Autodesk Inventor part; units mm, degrees
ref_plane "YZ Plane" through (0, 0, 0) normal (1, 0, 0) x (0, 1, 0)
ref_plane "XZ Plane" through (0, 0, 0) normal (0, 1, 0) x (-1, 0, 0)
ref_plane "XY Plane" through (0, 0, 0) normal (0, 0, 1) x (1, 0, 0)
sketch "Sketch1" plane through (0, 0, 0) normal (0, 0, 1) x (1, 0, 0)
  circle A0 centre (0, 0) radius 40
  circle A1 centre (0, 0) radius 41.5
  circle A2 centre (0, 0) radius 3.5
  circle A3 centre (0, 0) radius 5
  circle A4 centre (26, 0) radius 6.8
  circle A5 centre (26, 0) radius 7.8
  line L0 (0, 0) -> (43.8957, 0) construction
  line L1 (4.9183, 0.9) -> (18.2521, 0.9)
  line L2 (33.7479, 0.9) -> (39.9899, 0.9)
  line L3 (4.9183, -0.9) -> (18.2521, -0.9)
  line L4 (33.7479, -0.9) -> (39.9899, -0.9)
  line L5 (-4.9183, -0.9) -> (-18.2521, -0.9)
  line L6 (-4.9183, 0.9) -> (-18.2521, 0.9)
  circle A6 centre (-26, 0) radius 7.8
  circle A7 centre (-26, 0) radius 6.8
  line L7 (-33.7479, 0.9) -> (-39.9899, 0.9)
  line L8 (-33.7479, -0.9) -> (-39.9899, -0.9)
  line L9 (1.2333, -3.7857) -> (-1.2333, -3.7857)
  line L10 (-1.6333, -3.3857) -> (-1.6333, 3.3857)
  line L11 (-1.2333, 3.7857) -> (1.2333, 3.7857)
  line L12 (1.6333, 3.3857) -> (1.6333, -3.3857)
  line L13 (1.6333, -3.7857) -> (-1.6333, 3.7857) construction
  line L14 (-1.6333, -3.7857) -> (1.6333, 3.7857) construction
  arc A8 (-1.2333, 3.7857) -> (-1.6333, 3.3857) centre (-1.2333, 3.3857) ccw
  arc A9 (1.6333, 3.3857) -> (1.2333, 3.7857) centre (1.2333, 3.3857) ccw
  arc A10 (1.2333, -3.7857) -> (1.6333, -3.3857) centre (1.2333, -3.3857) ccw
  arc A11 (-1.6333, -3.3857) -> (-1.2333, -3.7857) centre (-1.2333, -3.3857) ccw
  line L15 (3.3857, -1.6333) -> (-3.3857, -1.6333)
  line L16 (-3.7857, -1.2333) -> (-3.7857, 1.2333)
  line L17 (-3.3857, 1.6333) -> (3.3857, 1.6333)
  line L18 (3.7857, 1.2333) -> (3.7857, -1.2333)
  line L19 (3.7857, -1.6333) -> (-3.7857, 1.6333) construction
  line L20 (-3.7857, -1.6333) -> (3.7857, 1.6333) construction
  arc A12 (-3.3857, 1.6333) -> (-3.7857, 1.2333) centre (-3.3857, 1.2333) ccw
  arc A13 (3.7857, 1.2333) -> (3.3857, 1.6333) centre (3.3857, 1.2333) ccw
  arc A14 (3.3857, -1.6333) -> (3.7857, -1.2333) centre (3.3857, -1.2333) ccw
  arc A15 (-3.7857, -1.2333) -> (-3.3857, -1.6333) centre (-3.3857, -1.2333) ccw
  point P0 (-4.9183, -0.9)
  point P1 (4.9183, -0.9)
  point P2 (-1.6333, -3.0955)
  point P3 (-1.6333, 3.0955)
  point P4 (1.6333, 3.0955)
  point P5 (1.6333, -3.0955)
  point P6 (-4.9183, 0.9)
  point P7 (-33.7479, 0.9)
  point P8 (-3.0955, -1.6333)
  point P9 (-3.0955, 1.6333)
  point P10 (3.0955, 1.6333)
  point P11 (3.0955, -1.6333)
  dimension "d0" = 80
  dimension "d3" = 10
  dimension "d1" = 83
  dimension "d2" = 7
  dimension "d4" = 13.6
  dimension "d5" = 26
  dimension "d6" = 15.6
  dimension "d10" = 0.9
  dimension "d11" = 0.9
  dimension "d14" = 360
  dimension "d16" = 7.5714
  dimension "d17" = 3.2667
  dimension "d18" = 0.4
  dimension "d29" = 7.5714
  dimension "d30" = 3.2667
  dimension "d31" = 0.4
extrude "Extrusion1" add sketch "Sketch1" along normal blind 5 contours A0 L4 A5 L2 | L7 A6 L8 A0 | A5 | A6 | A5 L3 A3 L1 | L6 A3 L5 A6 | A3 | A1
sketch "Sketch2" plane through (0, 0, 5) normal (0, 0, 1) x (1, 0, 0)
  arc A0 (33.7479, 0.9) -> (18.2521, 0.9) centre (26, 0) ccw
  circle A1 centre (26, 0) radius 7.7
  circle A2 centre (26, 0) radius 5.8
  arc A3 (18.2521, -0.9) -> (33.7479, -0.9) centre (26, 0) ccw
  circle A4 centre (-26, 0) radius 5.8
  circle A5 centre (-26, 0) radius 7.7
  point P0 (0, 0)
  point P1 (18.3528, 0.9)
  point P2 (33.6472, 0.9)
  point P3 (-18.2521, 0.9)
  point P4 (-33.7479, 0.9)
  point P5 (18.7723, -2.9327)
  dimension "d21" = 7.8
  dimension "d22" = 11.6
  dimension "d27" = 360
extrude "Extrusion2" add sketch "Sketch2" along normal blind 0.4
equation "\"d0\" = D_yttreRing_i"
equation "\"d3\" = D_axel + d_axelRing"
equation "\"d1\" = D_yttreRing_i + d_yttreRing"
equation "\"d2\" = D_axel"
equation "\"d4\" = D_magnet + d_toleransRing"
equation "\"d6\" = d_toleransRing + D_magnet + d_magnetHållarRing"
equation "\"d11\" = 0.5 * d_stöttor"
equation "\"d18\" = r_filletAxel"
equation "\"d31\" = r_filletAxel"
equation "\"d19\" = h_höjdMagnetRotor"
equation "\"d22\" = D_magnet - d_magnetSkydd"
equation "\"d23\" = h_magnetSkydd"
equation "\"D_yttreRing_i\" = 80"
equation "\"d_yttreRing\" = 3"
equation "\"D_magnet\" = 13"
equation "\"D_axel\" = 7"
equation "\"d_axelRing\" = 3"
equation "\"h_höjdMagnetRotor\" = 5"
equation "\"d_stöttor\" = 1.8"
equation "\"d_toleransRing\" = 0.6"
equation "\"d_magnetHållarRing\" = 2"
equation "\"l_magnetHållarRingFrånOrigo\" = 26"
equation "\"r_filletAxel\" = 0.4"
equation "\"h_magnetSkydd\" = 0.4"
equation "\"d_magnetSkydd\" = 1.4"
properties part number "Magnet_rotor_parametriserad_02"
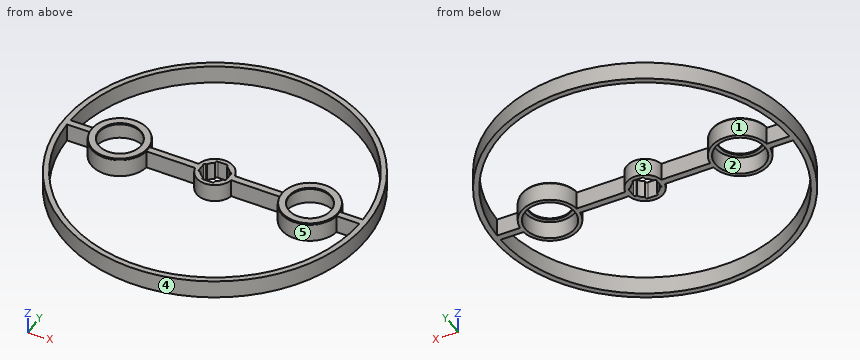
Read the model definition and answer for the solid it produces. Units are mm, in the model's axes. Face numbers are marked on the shaded views. A direction names the side the tool comes from. Round coordinates to 2 decimals unless told otherwise and drop trailing zeros. Order: outer loops, then holes, each group sorted by start corner. A loop starts at its lowest first (then second) coordinate and runs counter-clockwise, first axis right, second up.
1) The mould has two halves that part along X. Classify the marked faces 3, 4 and 5: released by +X, released by -X, zero draft, split by the parting line, or undercut.
2) For the marked faces 1 and 2, determine the directions among +Z, -Z, +X, -X, +Y, -Y from which every point of the face is accessible in a straight line to the end or side of a thin tool.
3) The part is cut by section C-C on x = 9. Write down the section's boundary in (y, z).
4) The part is cut by section B-B on y = -27. Write down the section's boundary in (x, z), plus the area to 3 significant figures.
5) Flat-ended cylindrical pins translate along their axes: pin 1 (1.5 mm diameter, centred on y = 26.5, z = 4.5, fed in from +X); pin 2 (2.5 mm diameter, centred on x = -8.5, z = 3.5, fed in from +Y); pin 3 (1.5 mm diameter, centred on x = 36.5, z = 3.5, fed in from +Y). Find the tip coordinate at first contact, or state that the pin passes through.
6) Straight lines are drawn through the part: L1, parallel to Y at x = -17.5, z = 1.25; L2, parallel to X at y = -7, z = 2.65; L3, parallel to Y at x = 26, z = 5.3. For each, find the intervals that lie inside material, in ascending order.
7) The part is cut by section D-D on y = -15. Write down the section's boundary in (x, z), plus the area to 3 significant figures.
8) The part is cut by section A-A on x = 0. Write down the section's boundary in (y, z), plus the area to 3 significant figures.
Resolved:
1. face 3: undercut
1. face 4: split by the parting line
1. face 5: undercut
2. face 1: +Z, -Z
2. face 2: -Z
3. outline: (-40.51, 0) - (-38.97, 0) - (-38.97, 5) - (-40.51, 5) - close; (-0.9, 0) - (0.9, 0) - (0.9, 5) - (-0.9, 5) - close; (38.97, 0) - (40.51, 0) - (40.51, 5) - (38.97, 5) - close
4. outline: (-31.52, 0) - (-29.51, 0) - (-29.51, 5) - (-31.52, 5) - close; (29.51, 0) - (31.52, 0) - (31.52, 5) - (29.51, 5) - close
4. area: 20.0 mm2
5. pin 1: stops at x = 32.55
5. pin 2: stops at y = 40.86
5. pin 3: stops at y = 21.08
6. L1: y = -37.63 to -35.97, -0.9 to 0.9, 35.97 to 37.63
6. L2: x = -40.91 to -39.38, -29.44 to -22.56, 22.56 to 29.44, 39.38 to 40.91
6. L3: y = -7.7 to -5.8, 5.8 to 7.7
7. outline: (-38.69, 0) - (-37.08, 0) - (-37.08, 5) - (-38.69, 5) - close; (37.08, 0) - (38.69, 0) - (38.69, 5) - (37.08, 5) - close
7. area: 16.1 mm2
8. outline: (-41.5, 0) - (-40, 0) - (-40, 5) - (-41.5, 5) - close; (-5, 0) - (-3.79, 0) - (-3.79, 5) - (-5, 5) - close; (3.79, 0) - (5, 0) - (5, 5) - (3.79, 5) - close; (40, 0) - (41.5, 0) - (41.5, 5) - (40, 5) - close
8. area: 27.1 mm2
